The figure shows three views and two pictorial views of one solid part (mm, origin at its lowest corner). Answer the questions. A direction names the side the tool comes from. Coordinates: 2 decimals unless noted, no trailing zeros. Loops run counter-clockwise (first coordinate to the right, second up) from the corner with the lowest first, then second, coordinate; pieces in that order, holes last. Notation, with made-up numbers: (13.25, -39) -> (61.25, -39) arc R11 cw to (61.25, -23) -> close; hole circle Ø6 at (1, 39.5). An arc over 180 degrees is marked (long way). Answer as a JSON object with one key per item and string values. Group by question number.
1) Consider probe 1 along Y at (x, z) = (18.5, 2.55); probe 2 along X at (y, z) = (3, 4); probe 3 along X at (y, z) = (1.75, 2.85). Determine where each line is inside the solid, lowest interval first. Write a range as [from, to].
2) Which of the six approach directions +Z, -Z, +X, -X, +Y, -Y give full straight-line access (tool end or side, diameter ignored) to the marked faces 5 and 6?
3) Section D-D, the plane x = 23 is taken. Give the vertices of the cut face in (y, z).
4) Section B-B, the plane x = 6.5 is taken. Give the vertices of the cut face in (y, z).
5) Flat-ended cylindrical pins translate along their axes: P1, Ø3, axis at x = 13.5, y = 4, coming from the -Z side; P2, Ø0.8, axis at x = 2, z = 3, coming from the +Y side; P3, Ø2.5, axis at x = 6.5, y = 2.75, coming from the +Z side. Find the tip coordinate at first contact, or state that the pin passes through.
6) Determine the mould class of the marked faces 1, 2, 3 and 4 for opening direction X: released by +X, released by -X, zero draft, split by the parting line, or undercut.
7) Section C-C, the plane z = 2.1 is taken. Count the separate pieces of the cut face and the enclosed holes in it, plus the area to 3 significant figures.
8) Section A-A, the plane y = 2.75 is taken. Give the vertices of the cut face in (x, z).
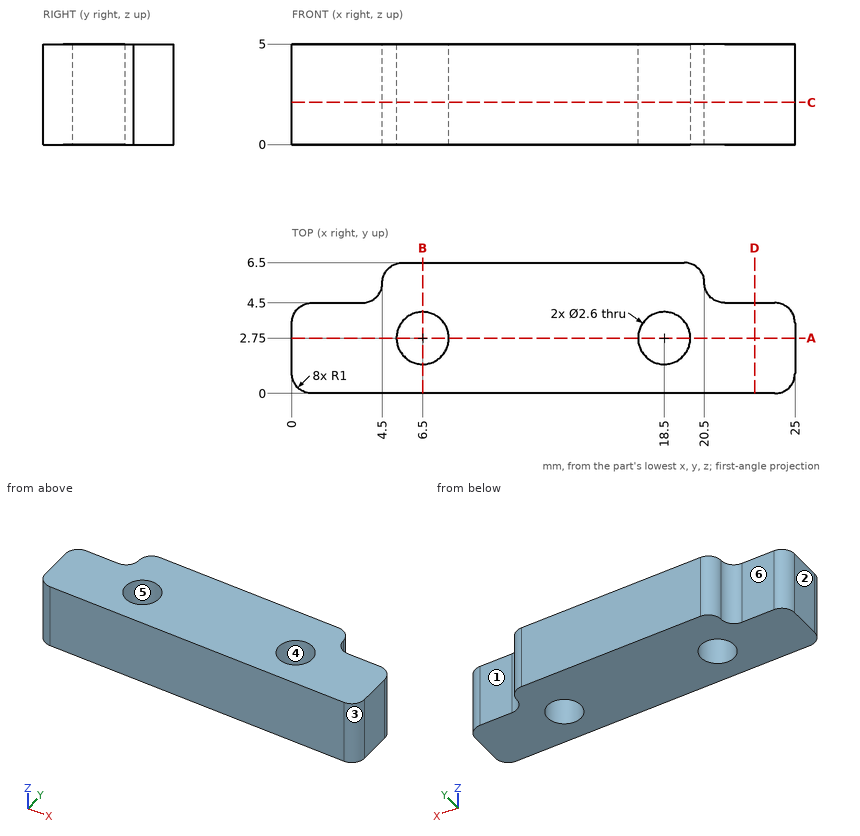
Determined:
{
 "1": {"probe 1": "[0, 1.45], [4.05, 6.5]", "probe 2": "[0, 5.22], [7.78, 17.22], [19.78, 25]", "probe 3": "[0, 5.67], [7.33, 17.67], [19.33, 25]"},
 "2": {"face 5": "+Z, -Z", "face 6": "+Z, -Z, -X, +Y"},
 "3": {"outline": "(0, 0) -> (4.5, 0) -> (4.5, 5) -> (0, 5) -> close"},
 "4": {"outline": "(0, 0) -> (1.45, 0) -> (1.45, 5) -> (0, 5) -> close; (4.05, 0) -> (6.5, 0) -> (6.5, 5) -> (4.05, 5) -> close"},
 "5": {"P1": "z = 0", "P2": "y = 4.5", "P3": "through"},
 "6": {"face 1": "zero draft", "face 2": "released by -X", "face 3": "released by +X", "face 4": "undercut"},
 "7": {"separate pieces": "1", "enclosed holes": "2", "area": "133 mm²"},
 "8": {"outline": "(0, 0) -> (5.2, 0) -> (5.2, 5) -> (0, 5) -> close; (7.8, 0) -> (17.2, 0) -> (17.2, 5) -> (7.8, 5) -> close; (19.8, 0) -> (25, 0) -> (25, 5) -> (19.8, 5) -> close"}
}
